Work out the finished part from the listing and answer in its coordinate system (mm). A direction names the side the tool comes from. Coordinates: 2 decimals unless noted, no trailing zeros. Order: outer loops, then holes, each group sorted by start corner. A loop starts at its lowest first (then second) coordinate and runs counter-clockwise, first axis right, second up. Notation, with made-up numbers: (-37.75, 8.5) - (0.25, 8.5) arc R23 ccw to (0.25, 18.5) - close; hole circle Ø9 at (20, 65.5). An arc over 180 degrees is marked (long way). Answer as a JSON object with one key per item and string values. Group by question number.
1) This flat-tipped pin is pushed along its axis until it touches: P1, Ø12, axis at x = -30.5, y = -6.5, coming from the -Z side. Where does it stop, or does it pass through?
2) Section B-B (z = 0.6) is taken. Count the separate pieces of the cut face and the enclosed holes in it, plus the area to 3 significant figures.
3) A tool of negligible diameter and unlimited length cuts with its end or side. For faces 5 (the face through (-18.5, -8, 1)), 6 (the face through (60.9, 18.23, 1.01)), from which of +Z, -Z, +X, -X, +Y, -Y can it reach the whole face along a straight path? Write none if from no direction.
4) Section A-A (x = -56.5) is taken. Give the vertices of the cut face in (y, z), plus the area to 3 significant figures.
5) The mould has two halves that part along Y. Classify faces 1 (the face through (19, -12, 1)), 2 (the face through (-8.5, -8, 1)), 3 (the face through (-61.5, 0, 1)), 4 (the face through (-60.93, 18.2, 1.01)): released by +Y, released by -Y, zero draft, split by the parting line, or undercut.
6) Find the intervals of material crossed by line 1 along Y through (x, z) = (-37.5, 1.5); line 2 along Y through (x, z) = (-56.5, 0.5); line 3 along X through (y, z) = (5.5, 1.2), in increasing order.
from build123d import *

# Parameters (mm, degrees)
SKETCH_1_W          = 123
SKETCH_1_H          = 37.6
EXTRUDE_1_DEPTH     = 2
SKETCH_2_R          = 1.55
CUT_EXTRUDE_1_DEPTH = 10
SKETCH_3_W          = 35
SKETCH_3_H          = 29.6
CUT_EXTRUDE_2_DEPTH = 10
FILLET_1_R          = 2
SKETCH_4_W          = 4
SKETCH_4_H          = 4
CUT_EXTRUDE_3_DEPTH = 10
FILLET_2_R          = 1.1
SKETCH_5_W          = 35
SKETCH_5_H          = 4
EXTRUDE_1_2_DEPTH   = 2
FILLET_3_R          = 2


with BuildPart() as part:
    # 草图1 → Extrude 1 (new body)
    with BuildSketch(Plane.XY):
        Rectangle(SKETCH_1_W, SKETCH_1_H)
    extrude(amount=EXTRUDE_1_DEPTH)

    # 草图2 → 切除-拉伸1 (cut)
    with BuildSketch(Plane.XY.offset(2)):
        with Locations((56.5, 15.8)):
            Circle(SKETCH_2_R)
        with Locations((58.5, -13.75)):
            Circle(SKETCH_2_R)
        with Locations((-56.5, 15.8)):
            Circle(SKETCH_2_R)
    extrude(amount=-CUT_EXTRUDE_1_DEPTH, mode=Mode.SUBTRACT)

    # 草图3 → 切除-拉伸2 (cut)
    with BuildSketch(Plane.XY.offset(2)):
        with Locations((-36, 0)):
            Rectangle(SKETCH_3_W, SKETCH_3_H)
    extrude(amount=-CUT_EXTRUDE_2_DEPTH, mode=Mode.SUBTRACT)

    # 圆角1
    fillet_1_edges = [part.edges().sort_by_distance(p)[0] for p in [
        (-18.5, 14.8, 1),
        (-18.5, -14.8, 1),
        (-53.5, -14.8, 1),
        (-53.5, 14.8, 1),
        (61.5, -18.8, 1),
        (-61.5, -18.8, 1),
        (-61.5, 18.8, 1),
        (61.5, 18.8, 1),
    ]]
    fillet(fillet_1_edges, radius=FILLET_1_R)

    # 草图4 → 切除-拉伸3 (cut)
    with BuildSketch(Plane.XY.offset(2)):
        Polygon((23, -9.986290852), (23, -14.8), (50.5, -14.8), (50.5, -2), (33.407936873, -2), align=None)
        Polygon((33.407936873, 2), (50.5, 2), (50.5, 14.8), (23, 14.8), (23, 9.986290852), align=None)
        Polygon((-8.5, 14.8), (-8.5, 2), (8.592063127, 2), (19, 9.986290852), (19, 14.8), align=None)
        Polygon((-8.5, -2), (-8.5, -14.8), (19, -14.8), (19, -9.986290852), (8.592063127, -2), align=None)
        Polygon((23, -2), (26.837218346, -2), (29.443669092, 0), (26.837218346, 2), (23, 2), align=None)
        Polygon((23, -2), (23, -4.944401196), (26.837218346, -2), align=None)
        Polygon((19, -2), (19, -4.944401196), (21, -6.479055172), (23, -4.944401196), (23, -2), align=None)
        Polygon((15.162781654, -2), (19, -4.944401196), (19, -2), align=None)
        Polygon((12.556330908, 0), (15.162781654, -2), (19, -2), (19, 2), (15.162781654, 2), align=None)
        Polygon((19, 4.944401196), (15.162781654, 2), (19, 2), align=None)
        Polygon((19, 4.944401196), (19, 2), (23, 2), (23, 4.944401196), (21, 6.479055172), align=None)
        Polygon((23, 4.944401196), (23, 2), (26.837218346, 2), align=None)
        with Locations((21, 0)):
            Rectangle(SKETCH_4_W, SKETCH_4_H)
    extrude(amount=-CUT_EXTRUDE_3_DEPTH, mode=Mode.SUBTRACT)

    # 圆角2
    fillet_2_edges = [part.edges().sort_by_distance(p)[0] for p in [
        (33.407936873, 2, 1),
        (23, 9.986290852, 1),
        (23, 14.8, 1),
        (50.5, 14.8, 1),
        (50.5, 2, 1),
        (-8.5, 2, 1),
        (-8.5, 14.8, 1),
        (19, 14.8, 1),
        (19, 9.986290852, 1),
        (8.592063127, 2, 1),
        (21, 6.479055172, 1),
        (29.443669092, 0, 1),
        (21, -6.479055172, 1),
        (12.556330908, 0, 1),
        (-8.5, -2, 1),
        (8.592063127, -2, 1),
        (19, -9.986290852, 1),
        (19, -14.8, 1),
        (-8.5, -14.8, 1),
        (23, -9.986290852, 1),
        (33.407936873, -2, 1),
        (50.5, -2, 1),
        (50.5, -14.8, 1),
        (23, -14.8, 1),
    ]]
    fillet(fillet_2_edges, radius=FILLET_2_R)

    # 草图5 → Extrude 1 2 (add)
    with BuildSketch(Plane.XY.offset(2)):
        with Locations((-36, 0)):
            Rectangle(SKETCH_5_W, SKETCH_5_H)
    extrude(amount=-EXTRUDE_1_2_DEPTH)

    # 圆角3
    fillet_3_edges = [part.edges().sort_by_distance(p)[0] for p in [
        (-53.5, 2, 1),
        (-18.5, 2, 1),
        (-18.5, -2, 1),
        (-53.5, -2, 1),
    ]]
    fillet(fillet_3_edges, radius=FILLET_3_R)


solid = part.part
Report:
{
 "1": {"P1": "stops at z = 0"},
 "2": {"separate pieces": "1", "enclosed holes": "10", "area": "2,360 mm²"},
 "3": {"face 5": "+Z, -Z", "face 6": "+Z, -Z, +X, +Y"},
 "4": {"outline": "(-18.8, 0) - (14.25, 0) - (14.25, 2) - (-18.8, 2) - close; (17.35, 0) - (18.8, 0) - (18.8, 2) - (17.35, 2) - close", "area": "69.0 mm²"},
 "5": {"face 1": "undercut", "face 2": "undercut", "face 3": "zero draft", "face 4": "released by +Y"},
 "6": {"line 1": "y = -18.8 to -14.8, -2 to 2, 14.8 to 18.8", "line 2": "y = -18.8 to 14.25, 17.35 to 18.8", "line 3": "x = -61.5 to -53.5, -18.5 to -8.5, 13.15 to 19.72, 22.28 to 28.85, 50.5 to 61.5"}
}
